from build123d import *

# Parameters (mm, degrees)
SKETCH1_R            = 1.6
BOSS_EXTRUDE1_DEPTH  = 4
CUT_EXTRUDE1_DEPTH   = 2
CUT_EXTRUDE2_DEPTH   = 1.5
SKETCH4_R            = 1.5
CUT_EXTRUDE3_DEPTH   = 52.039200621
BOSS_EXTRUDE2_START  = 1.5
SKETCH5_R            = 4
SKETCH5_R_2          = 1.5
BOSS_EXTRUDE2_DEPTH  = 1.5
FILLET1_R            = 2
FILLET1_OF_MIRROR1_R = 2
MIRROR2_3_OUTLINE_W  = 1.5
MIRROR2_3_OUTLINE_H  = 2
MIRROR2_4_OUTLINE_W  = 1.5
MIRROR2_4_OUTLINE_H  = 2


# Read off the part's stored shape, not the designer's step: Mirror2
with BuildPart() as part:
    # Sketch1 → Boss-Extrude1 (new body)
    with BuildSketch(Plane.XY):
        Polygon((-35, 12.5), (-36.062445841, 23.334523779), (-23.334523779, 36.062445841), (-12.5, 35), (12.5, 35), (23.334523779, 36.062445841), (36.062445841, 23.334523779), (35, 12.5), (35, -12.5), (36.062445841, -23.334523779), (23.334523779, -36.062445841), (12.5, -35), (-12.5, -35), (-23.334523779, -36.062445841), (-36.062445841, -23.334523779), (-35, -12.5), align=None)
        with Locations((-22.627416998, 31.112698372)):
            Circle(SKETCH1_R, mode=Mode.SUBTRACT)
        with Locations((-31.112698372, 22.627416998)):
            Circle(SKETCH1_R, mode=Mode.SUBTRACT)
        with Locations((-31.112698372, -22.627416998)):
            Circle(SKETCH1_R, mode=Mode.SUBTRACT)
        with Locations((-22.627416998, -31.112698372)):
            Circle(SKETCH1_R, mode=Mode.SUBTRACT)
        with Locations((22.627416998, -31.112698372)):
            Circle(SKETCH1_R, mode=Mode.SUBTRACT)
        with Locations((31.112698372, -22.627416998)):
            Circle(SKETCH1_R, mode=Mode.SUBTRACT)
        with Locations((31.112698372, 22.627416998)):
            Circle(SKETCH1_R, mode=Mode.SUBTRACT)
        with Locations((22.627416998, 31.112698372)):
            Circle(SKETCH1_R, mode=Mode.SUBTRACT)
    extrude(amount=BOSS_EXTRUDE1_DEPTH)

    # Sketch2 → Cut-Extrude1 (cut)
    with BuildSketch(Plane(origin=(0, 0, 0), x_dir=(-1, 0, 0), z_dir=(0, 0, -1))):
        Polygon((-17.669047558, 29), (17.669047558, 29), (29, 17.669047558), (29, -17.669047558), (17.669047558, -29), (-17.669047558, -29), (-29, -17.669047558), (-29, 17.669047558), align=None)
    extrude(amount=-CUT_EXTRUDE1_DEPTH, mode=Mode.SUBTRACT)

    # Sketch3 → Cut-Extrude2 (cut)
    with BuildSketch(Plane(origin=(0, 0, 2), x_dir=(-1, 0, 0), z_dir=(0, 0, -1))):
        with BuildLine():
            Line((-24.58547182, -11.125115865), (-16.58547182, -6.847712761))
            ThreePointArc((-16.58547182, -6.847712761), (-15.426715665, -5.744273519), (-15, -4.202129644))
            Line((-15, -4.202129644), (-15, 4.202129644))
            ThreePointArc((-15, 4.202129644), (-15.426715665, 5.744273519), (-16.58547182, 6.847712761))
            Line((-16.58547182, 6.847712761), (-24.58547182, 11.125115865))
            ThreePointArc((-24.58547182, 11.125115865), (-27.542143875, 11.052817083), (-29, 8.479532748))
            Line((-29, 8.479532748), (-29, -8.479532748))
            ThreePointArc((-29, -8.479532748), (-27.542143875, -11.052817083), (-24.58547182, -11.125115865))
        make_face()
        with BuildLine():
            Line((6.847712761, 16.58547182), (11.125115865, 24.58547182))
            ThreePointArc((11.125115865, 24.58547182), (11.052817083, 27.542143875), (8.479532748, 29))
            Line((8.479532748, 29), (-8.479532748, 29))
            ThreePointArc((-8.479532748, 29), (-11.052817083, 27.542143875), (-11.125115865, 24.58547182))
            Line((-11.125115865, 24.58547182), (-6.847712761, 16.58547182))
            ThreePointArc((-6.847712761, 16.58547182), (-5.744273519, 15.426715665), (-4.202129644, 15))
            Line((-4.202129644, 15), (4.202129644, 15))
            ThreePointArc((4.202129644, 15), (5.744273519, 15.426715665), (6.847712761, 16.58547182))
        make_face()
        with BuildLine():
            Line((16.58547182, -6.847712761), (24.58547182, -11.125115865))
            ThreePointArc((24.58547182, -11.125115865), (27.542143875, -11.052817083), (29, -8.479532748))
            Line((29, -8.479532748), (29, 8.479532748))
            ThreePointArc((29, 8.479532748), (27.542143875, 11.052817083), (24.58547182, 11.125115865))
            Line((24.58547182, 11.125115865), (16.58547182, 6.847712761))
            ThreePointArc((16.58547182, 6.847712761), (15.426715665, 5.744273519), (15, 4.202129644))
            Line((15, 4.202129644), (15, -4.202129644))
            ThreePointArc((15, -4.202129644), (15.426715665, -5.744273519), (16.58547182, -6.847712761))
        make_face()
        with BuildLine():
            Line((-6.847712761, -16.58547182), (-11.125115865, -24.58547182))
            ThreePointArc((-11.125115865, -24.58547182), (-11.052817083, -27.542143875), (-8.479532748, -29))
            Line((-8.479532748, -29), (8.479532748, -29))
            ThreePointArc((8.479532748, -29), (11.052817083, -27.542143875), (11.125115865, -24.58547182))
            Line((11.125115865, -24.58547182), (6.847712761, -16.58547182))
            ThreePointArc((6.847712761, -16.58547182), (5.744273519, -15.426715665), (4.202129644, -15))
            Line((4.202129644, -15), (-4.202129644, -15))
            ThreePointArc((-4.202129644, -15), (-5.744273519, -15.426715665), (-6.847712761, -16.58547182))
        make_face()
    extrude(amount=-CUT_EXTRUDE2_DEPTH, mode=Mode.SUBTRACT)

    # Sketch4 → Cut-Extrude3 (cut, through all)
    with BuildSketch(Plane(origin=(0, 0, 2), x_dir=(-1, 0, 0), z_dir=(0, 0, -1))):
        with Locations((15.25, 15.25)):
            Circle(SKETCH4_R)
    cut_extrude3 = extrude(amount=-CUT_EXTRUDE3_DEPTH, mode=Mode.SUBTRACT)

    # Sketch5 → Boss-Extrude2 (add)
    with BuildSketch(Plane(origin=(0, 0, 2), x_dir=(-1, 0, 0), z_dir=(0, 0, -1)).offset(BOSS_EXTRUDE2_START)):
        with Locations(Location((15.25, 15.25, 0), (0, 0, 180))):
            Circle(SKETCH5_R)
        with Locations((15.25, 15.25)):
            Circle(SKETCH5_R_2, mode=Mode.SUBTRACT)
    boss_extrude2 = extrude(amount=-BOSS_EXTRUDE2_DEPTH)

    # Fillet1
    # the kernel refuses this fillet: 2 mm, written as the material it adds along each edge
    with BuildSketch(Plane(origin=(-15.25, 15.25, 2), x_dir=(1, 0, 0), z_dir=(0, 1, 0))) as fillet1_piece_1:
        with BuildLine():
            CenterArc((5.936491673, 2), FILLET1_R, 194.477512186, 75.522487814)
            Line((5.936491673, 0), (5.936491673, -0.04))
            Line((5.936491673, -0.04), (4, -0.04))
            Line((4, -0.04), (3.96, 0))
            ThreePointArc((3.96, 0), (3.96, 0.75), (3.961270167, 1.49))
            Line((3.961270167, 1.49), (4, 1.5))
        make_face()
    revolve(axis=Axis((-15.25, 15.25, 2), (0, 0, -1)))

    # Mirror1: Cut-Extrude3, Boss-Extrude2 across plane
    add(cut_extrude3.mirror(Plane(origin=(0, 0, 0), x_dir=(0, 0, 1), z_dir=(1, 0, 0))), mode=Mode.SUBTRACT)
    add(boss_extrude2.mirror(Plane(origin=(0, 0, 0), x_dir=(0, 0, 1), z_dir=(1, 0, 0))))

    # Fillet1 of Mirror1
    # the kernel refuses this fillet: 2 mm, written as the material it adds along each edge
    with BuildSketch(Plane(origin=(15.25, 15.25, 2), x_dir=(-1, 0, 0), z_dir=(0, 1, 0))) as fillet1_of_mirror1_piece_1:
        with BuildLine():
            CenterArc((5.936491673, -2), FILLET1_OF_MIRROR1_R, 90, 75.522487814)
            Line((5.936491673, 0), (5.936491673, 0.04))
            Line((5.936491673, 0.04), (4, 0.04))
            Line((4, 0.04), (3.96, 0))
            ThreePointArc((3.96, 0), (3.96, -0.75), (3.961270167, -1.49))
            Line((3.961270167, -1.49), (4, -1.5))
        make_face()
    revolve(axis=Axis((15.25, 15.25, 2), (0, 0, 1)))

    # Mirror2 outline → Mirror2 (revolve)
    with BuildSketch(Plane(origin=(15.25, -15.25, 0), x_dir=(1, 0, 0), z_dir=(0, -1, 0))):
        with BuildLine():
            Line((1.5, 2), (1.5, 0.5))
            Line((1.5, 0.5), (4, 0.5))
            ThreePointArc((4, 0.5), (4.711746802, 1.58113883), (5.936491673, 2))
            Line((5.936491673, 2), (1.5, 2))
        make_face()
    revolve(axis=Axis((15.25, -15.25, 0), (0, 0, 1)))

    # Mirror2 2 outline → Mirror2 2 (revolve)
    with BuildSketch(Plane(origin=(-15.25, -15.25, 0), x_dir=(1, 0, 0), z_dir=(0, -1, 0))):
        with BuildLine():
            Line((1.5, 2), (1.5, 0.5))
            Line((1.5, 0.5), (4, 0.5))
            ThreePointArc((4, 0.5), (4.711746802, 1.58113883), (5.936491673, 2))
            Line((5.936491673, 2), (1.5, 2))
        make_face()
    revolve(axis=Axis((-15.25, -15.25, 0), (0, 0, 1)))

    # Mirror2 3 outline → Mirror2 3 (revolve, cut)
    with BuildSketch(Plane(origin=(15.25, -15.25, 0), x_dir=(1, 0, 0), z_dir=(0, -1, 0))):
        with Locations((0.75, 3)):
            Rectangle(MIRROR2_3_OUTLINE_W, MIRROR2_3_OUTLINE_H)
    revolve(axis=Axis((15.25, -15.25, 0), (0, 0, 1)), mode=Mode.SUBTRACT)

    # Mirror2 4 outline → Mirror2 4 (revolve, cut)
    with BuildSketch(Plane(origin=(-15.25, -15.25, 0), x_dir=(1, 0, 0), z_dir=(0, -1, 0))):
        with Locations((0.75, 3)):
            Rectangle(MIRROR2_4_OUTLINE_W, MIRROR2_4_OUTLINE_H)
    revolve(axis=Axis((-15.25, -15.25, 0), (0, 0, 1)), mode=Mode.SUBTRACT)


solid = part.part
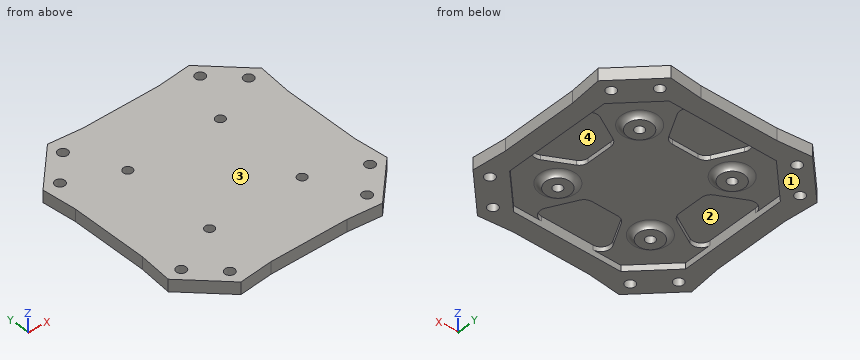
Here's how the part is built. I have some questions about the finished solid (model axes, mm). Face numbers are marked on the shaded views. A direction names the side the tool comes from. Give positions to 0.01 mm unless a question says otherwise; leave off trailing zeros. Order: outer loops, then holes, each group sorted by start corner. A loop starts at its lowest first (then second) coordinate and runs counter-clockwise, first axis right, second up. Notation, with made-up numbers: (70.25, 82) -> (113.25, 82) arc R13 ccw to (113.25, 104) -> close; hole circle Ø5 at (-23, 56.5). An arc over 180 degrees is marked (long way). Use a Markdown table: item, result. Add a question column.
Item 1: Imagine slicing it at C-C on z = 1.2. Give the number of separate pieces and of enclosed holes in the cut face, plus the area to 3 significant figures.
Item 2: Imagine slicing it at A-A on y = 2. Please give me the cut outline in (x, z).
Item 3: Will these pins go through, and if not, where does the flat tip stop? pin 1 (9 mm diameter, centred on x = 15.5, y = -16, fed in from -Z); pin 2 (2 mm diameter, centred on x = -1, z = 1, fed in from +Y); pin 3 (2 mm diameter, centred on y = 6.5, z = 1, fed in from -X).
Item 4: For the marked faces 3 and 4, which set-ups out of +Z, -Z, +X, -X, +Y, -Y let a thin tool reach every point of the face, with its end or its side?
Item 5: I need wall thicknesses on line 1 (X direction, y = -8.5, z = 1.25); line 2 (X direction, y = 22, z = 1.8). Which ranges of each line are inside material? Lowest first, please.
Item 6: If we mould it in two halves opening along Y, with no side actions, what happens to the marked faces 1 and 2? For each: pulls with the +Y half, pulls with the -Y half, needs draft (parallel to the pull), parting line crosses it, or undercut.
Data:
| question | item | result |
|---|---|---|
| 1 | separate pieces | 5 |
| 1 | enclosed holes | 13 |
| 1 | area | 1,760 mm² |
| 2 | outline | (-35, 0) -> (-29, 0) -> (-29, 3.5) -> (-15, 3.5) -> (-15, 2) -> (15, 2) -> (15, 3.5) -> (29, 3.5) -> (29, 0) -> (35, 0) -> (35, 4) -> (-35, 4) -> close |
| 3 | pin 1 | stops at z = 0.5 |
| 3 | pin 2 | stops at y = 35 |
| 3 | pin 3 | stops at x = -35 |
| 4 | face 3 | +Z, +X, -X, +Y, -Y |
| 4 | face 4 | -Z |
| 5 | line 1 | x = -35 to -29, 29 to 35 |
| 5 | line 2 | x = -35.93 to -32.58, -29.64 to -24.67, 24.67 to 29.64, 32.58 to 35.93 |
| 6 | face 1 | needs draft |
| 6 | face 2 | undercut |
